CAD build for the part. Positions are in the model's coordinates, mm. A direction names the side the tool comes from. Give positions to 0.01 mm unless a question says otherwise; leave off trailing zeros. Order: outer loops, then holes, each group sorted by start corner. A loop starts at its lowest first (then second) coordinate and runs counter-clockwise, first axis right, second up.
Item 1: Flat gauge pins, fed straight in: P1, Ø10, axis at x = 200, z = 0, coming from the +Y side; P2, Ø3, axis at x = 106, y = 11, coming from the -Z side; P3, Ø1.7, axis at x = 76, y = 11.5, coming from the -Z side. Where does each tip first touch, or does it go through?
Item 2: Which spindle directions (+Z, -Z, +X, -X, +Y, -Y) get a long thin tool onto all of the face, cutting with end or side? Do faces 1 (the flat face through (108, 4, 11.5)), 2 (the flat face through (220, 11, 0)), 3 (the flat face through (108, 22, 0)), 4 (the flat face through (108.5, 8.1, -9.6)), 5 (the flat face through (140, 13, 4)). Say none if no direction does.
Item 3: Wall check: L1, parallel to X at y = 9.5, z = 0; L2, parallel to X at y = 18.5, z = 0; L3, parallel to Z at x = 200, y = 10. Give the ranges that are in metal, low to high.
Item 4: Band-saw the part on B-B on x = 52. Give the cut face in (y, z).
Item 5: Band-saw the part on C-C on z = 0. Count the separate pieces of the cut face and the enclosed holes in it, plus the area to 3 significant figures.
Item 6: Two-plate mould, pull along Y, no slides. Class faces 6 (the flat face through (108, 12, 7.7)), 7 (the flat face through (108, 0, 0)), 8 (the cylindrical face through (145.453, 17.563, -0.716)): released by +Y, released by -Y, zero draft, split by the parting line, or undercut.
```python
from build123d import *

# Parameters (mm, degrees)
BOSS_EXTRUDE1_DEPTH   = 220
BOLT_HOLE_D           = 7
BOLT_HOLE_CBORE_D     = 11
BOLT_HOLE_CBORE_DEPTH = 9
BOLT_PATTERN_COUNT    = 4
BOLT_PATTERN_PITCH    = 60


with BuildPart() as part:
    # Sketch1 → Boss-Extrude1 (new body)
    with BuildSketch(Plane(origin=(0, 0, 0), x_dir=(0, 0, -1), z_dir=(1, 0, 0))):
        with BuildLine():
            Line((-10, 0), (10, 0))
            Line((10, 0), (11.5, 1.5))
            Line((11.5, 1.5), (11.5, 6.2))
            Line((11.5, 6.2), (7.7, 10))
            Line((7.7, 10), (7.7, 13.38))
            Line((7.7, 13.38), (8.93, 14.61))
            ThreePointArc((8.93, 14.61), (9.671019844, 16.398980156), (11.46, 17.14))
            Line((11.46, 17.14), (11.68, 17.36))
            Line((11.68, 17.36), (11.68, 19.38))
            Line((11.68, 19.38), (11.47, 19.59))
            ThreePointArc((11.47, 19.59), (10.062857505, 20.172857505), (9.48, 21.58))
            Line((9.48, 21.58), (9.06, 22))
            Line((9.06, 22), (-9.06, 22))
            Line((-9.06, 22), (-9.48, 21.58))
            ThreePointArc((-9.48, 21.58), (-10.062857505, 20.172857505), (-11.47, 19.59))
            Line((-11.47, 19.59), (-11.68, 19.38))
            Line((-11.68, 19.38), (-11.68, 17.36))
            Line((-11.68, 17.36), (-11.46, 17.14))
            ThreePointArc((-11.46, 17.14), (-9.671019844, 16.398980156), (-8.93, 14.61))
            Line((-8.93, 14.61), (-7.7, 13.38))
            Line((-7.7, 13.38), (-7.7, 10))
            Line((-7.7, 10), (-11.5, 6.2))
            Line((-11.5, 6.2), (-11.5, 1.5))
            Line((-11.5, 1.5), (-10, 0))
        make_face()
    extrude(amount=BOSS_EXTRUDE1_DEPTH)

    # Bolt Hole (through all)
    with Locations(Plane(origin=(20, 22, 0), x_dir=(0, 0, 1), z_dir=(0, 1, 0))):
        with Locations((0, 0)):
            bolt_hole = CounterBoreHole(BOLT_HOLE_D / 2, BOLT_HOLE_CBORE_D / 2, BOLT_HOLE_CBORE_DEPTH)

    # Bolt Pattern: Bolt Hole ×4
    with Locations(*[(i * BOLT_PATTERN_PITCH, 0, 0) for i in range(1, BOLT_PATTERN_COUNT)]):
        add(bolt_hole, mode=Mode.SUBTRACT)


solid = part.part
```
The answers:
1. P1: stops at y = 13
1. P2: stops at z = -8.2
1. P3: stops at z = -7.7
2. face 1: +Z, +X, -X, -Y
2. face 2: +Z, -Z, +X, +Y, -Y
2. face 3: +Z, -Z, +X, -X, +Y
2. face 4: -Z, +X, -X
2. face 5: +Y
3. L1: x = 0 to 16.5, 23.5 to 76.5, 83.5 to 136.5, 143.5 to 196.5, 203.5 to 220
3. L2: x = 0 to 14.5, 25.5 to 74.5, 85.5 to 134.5, 145.5 to 194.5, 205.5 to 220
3. L3: z = -7.7 to -3.5, 3.5 to 7.7
4. outline: (0, -10) - (1.5, -11.5) - (6.2, -11.5) - (10, -7.7) - (13.38, -7.7) - (14.61, -8.93) arc R2.53 cw to (17.14, -11.46) - (17.36, -11.68) - (19.38, -11.68) - (19.59, -11.47) arc R1.99 cw to (21.58, -9.48) - (22, -9.06) - (22, 9.06) - (21.58, 9.48) arc R1.99 cw to (19.59, 11.47) - (19.38, 11.68) - (17.36, 11.68) - (17.14, 11.46) arc R2.53 cw to (14.61, 8.93) - (13.38, 7.7) - (10, 7.7) - (6.2, 11.5) - (1.5, 11.5) - (0, 10) - close
5. separate pieces: 5
5. enclosed holes: 0
5. area: 4,080 mm2
6. face 6: undercut
6. face 7: released by -Y
6. face 8: zero draft
